Source: three-view drawing plus pictorial views. Frame: mm from the lowest corner of the part. Give positions to 0.01 mm unless a question says otherwise; leave off trailing zeros. Order: outer loops, then holes, each group sorted by start corner. A loop starts at its lowest first (then second) coordinate and runs counter-clockwise, first axis right, second up. Notation, with made-up numbers: (78.25, -35) -> (96.25, -35) arc R27 ccw to (96.25, 1) -> close; hole circle Ø1 at (13.25, 67.5). An arc over 180 degrees is marked (long way). One line per question, with ' | ' between items.
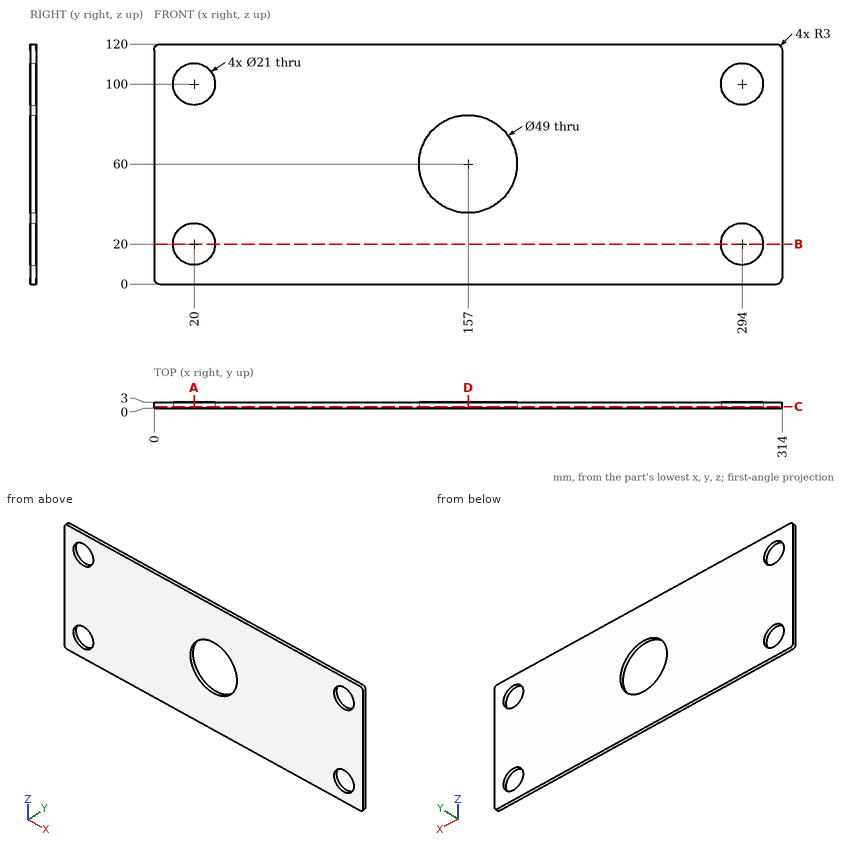
1) Section D-D on x = 157. Return loops of the section in (y, z).
Check result:
outline: (0, 0) -> (3, 0) -> (3, 35.5) -> (0, 35.5) -> close; (0, 84.5) -> (3, 84.5) -> (3, 120) -> (0, 120) -> close
2) Contact query for a flat-ended pin moving along its axis: pin 1 Ø12.5 at (x, z) = (294, 100) entering from +Y. Output: stop coordinate, or through.
Check result:
pin 1: passes through
3) Section B-B on z = 20. Return loops of the section in (x, y).
Check result:
outline: (0, 0) -> (9.5, 0) -> (9.5, 3) -> (0, 3) -> close; (30.5, 0) -> (283.5, 0) -> (283.5, 3) -> (30.5, 3) -> close; (304.5, 0) -> (314, 0) -> (314, 3) -> (304.5, 3) -> close
4) Section A-A on x = 20. Return loops of the section in (y, z), plus the area to 3 significant figures.
Check result:
outline: (0, 0) -> (3, 0) -> (3, 9.5) -> (0, 9.5) -> close; (0, 30.5) -> (3, 30.5) -> (3, 89.5) -> (0, 89.5) -> close; (0, 110.5) -> (3, 110.5) -> (3, 120) -> (0, 120) -> close | area: 234 mm^2
5) Material intervals for probe 1 along Z at (x, y) = (294, 1.9); probe 2 along X at (y, z) = (1.6, 100); probe 3 along Z at (x, y) = (300, 2.4), sorted ascending. Write a range as from..to.
Check result:
probe 1: z = 0..9.5, 30.5..89.5, 110.5..120 | probe 2: x = 0..9.5, 30.5..283.5, 304.5..314 | probe 3: z = 0..11.38, 28.62..91.38, 108.62..120
6) Section C-C on y = 0.65. Return loops of the section in (x, z), plus the area to 3 significant figures.
Check result:
outline: (0, 3) arc R3 ccw to (3, 0) -> (311, 0) arc R3 ccw to (314, 3) -> (314, 117) arc R3 ccw to (311, 120) -> (3, 120) arc R3 ccw to (0, 117) -> close; hole circle Ø21 at (20, 20); hole circle Ø21 at (20, 100); hole circle Ø49 at (157, 60); hole circle Ø21 at (294, 20); hole circle Ø21 at (294, 100) | area: 34,400 mm^2
